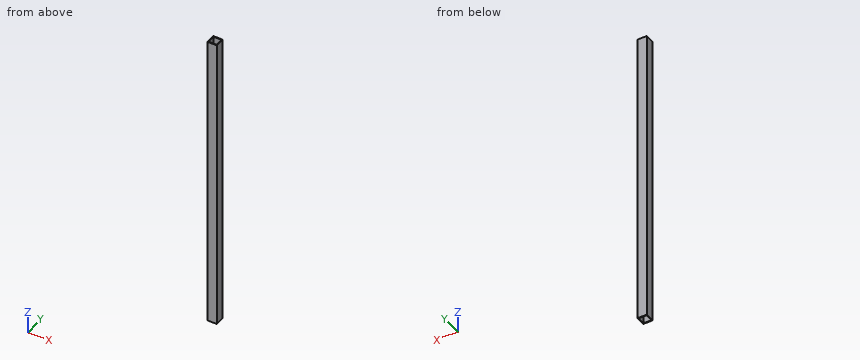
Autodesk Inventor part; units mm, degrees
ref_plane "Start Plane" through (0, 0, -19.05) normal (0, 0, 1) x (1, 0, 0)
ref_plane "End Plane" through (0, 0, 1187.45) normal (0, 0, 1) x (1, 0, 0)
ref_plane "Work Plane5" through (685.8, -19.05, -19.05) normal (0, 0, -1) x (-1, 0, 0)
ref_plane "Start Plane" through (0, 0, -19.05) normal (0, 0, 1) x (1, 0, 0)
ref_plane "End Plane" through (0, 0, 1187.45) normal (0, 0, 1) x (1, 0, 0)
sketch "Sketch" plane through (0, 0, 0) normal (0, 0, 1) x (1, 0, 0)
  line L0 (-19.05, 19.05) -> (19.05, 19.05)
  line L1 (19.05, 19.05) -> (19.05, -19.05)
  line L2 (19.05, -19.05) -> (-19.05, -19.05)
  line L3 (-19.05, -19.05) -> (-19.05, 19.05)
  line L4 (15.875, 15.875) -> (-15.875, 15.875)
  line L5 (-15.875, 15.875) -> (-15.875, -15.875)
  line L6 (-15.875, -15.875) -> (15.875, -15.875)
  line L7 (15.875, -15.875) -> (15.875, 15.875)
  point P0 (0, 0)
  point P1 (0, 19.05)
  point P2 (-19.05, 0)
  dimension "width" = 38.1
  dimension "d1" = 3.175
extrude "Body" add sketch "Sketch" along normal up to surface (1206.5 mm away) from surface at -19.05
sketch "Sketch4" plane through (0, 0, 0) normal (0, 0, 1) x (1, 0, 0)
  line L0 (0, 0) -> (10, 0)
ref_plane "Work Plane4" through (0, 0, 0) normal (0, -1, 0) x (1, 0, 0)
sketch "Sketch5" plane through (0, 0, 0) normal (0, -1, 0) x (1, 0, 0)
  line L0 (-2, -19.05) -> (12, -19.05)
  line L1 (-2, 1187.45) -> (12, 1187.45)
  dimension "d9" = 1206.5
ref_plane "Work Plane5" through (685.8, -19.05, -19.05) normal (0, 0, -1) x (-1, 0, 0)
split "Split1" plane through (685.8, -19.05, -19.05) removes the side toward (0, 0, -1)
ref_plane "Work Plane6" through (0, -19.05, 1187.45) normal (0, 0, 1) x (1, 0, 0)
split "Split2" plane through (0, -19.05, 1187.45) removes the side toward (0, 0, 1)
equation "\"G_OFFSET_START\" = 19.05"
equation "\"G_OFFSET_END\" = 19.05"
equation "\"d4\" = -G_OFFSET_START"
equation "\"d5\" = length + G_OFFSET_END"
equation "\"G_L\" = 1168.4"
properties part number "1.5x1.5x.125 Tube" material "Aluminum-6061"
The model under review builds one solid part; all positions refer to its coordinate system, in mm. Round coordinates to 2 decimals unless told otherwise and drop trailing zeros. Write each loop counter-clockwise with the first axis right and the second up, starting at its lowest first coordinate (ties: lowest second). Pieces come first, ordered by that corner, then holes. Notation, with made-up numbers: (-23, 35) -> (18, 35) arc R15 cw to (18, 47) -> close; hole circle Ø2 at (79, 74.25). An arc over 180 degrees is marked (long way). Use CSV: the item, a comma, the result in double quotes.
Q1. Consider section C-C (z = 259). Give the boundary of the cut face in (x, y) (3 decimals), then the cut area to 3 significant figures.
Checks:
outline,"(-19.05, -19.05) -> (19.05, -19.05) -> (19.05, 19.05) -> (-19.05, 19.05) -> close; hole (-15.875, -15.875) -> (15.875, -15.875) -> (15.875, 15.875) -> (-15.875, 15.875) -> close"
area,"444 mm²"
Q2. Consider section A-A (x = -3.5). Give the boundary of the cut face in (y, z) (3 decimals), then the cut area to 3 significant figures.
Checks:
outline,"(-19.05, -19.05) -> (-15.875, -19.05) -> (-15.875, 1187.45) -> (-19.05, 1187.45) -> close; (15.875, -19.05) -> (19.05, -19.05) -> (19.05, 1187.45) -> (15.875, 1187.45) -> close"
area,"7,660 mm²"
Q3. For pin 1 Ø8 at (x, y) = (-9.5, -1) entering from +Z, flat-tipped, find the tip position at first contact; note if it passes through.
Checks:
pin 1,"through"
Q4. To check wall thickness, follow probe 1 along Y at (x, z) = (-3.5, 548) (3 decimals). State the ranges of the line that lie inside material, in increasing order. Write a range as [from, to].
Checks:
probe 1,"[-19.05, -15.875], [15.875, 19.05]"
